from build123d import *

# Parameters (mm, degrees)
ESQUISSE1_R                  = 125
ESQUISSE1_W                  = 25
ESQUISSE1_H                  = 60
BOSS_EXTRU_1_DEPTH           = 5
ESQUISSE2_W                  = 5
ESQUISSE2_H                  = 30
BOSS_EXTRU_2_DEPTH           = 45
CONG_1_R                     = 15
ESQUISSE3_R                  = 6
ESQUISSE3_R_2                = 1.25
ENL_V_MAT_EXTRU_1_DEPTH      = 50
R_P_TITION_CIRCULAIRE1_COUNT = 3
ESQUISSE7_W                  = 24
ESQUISSE7_H                  = 37
BOSS_EXTRU_4_DEPTH           = 4.1
ESQUISSE8_R                  = 3
ENL_V_MAT_EXTRU_2_DEPTH      = 183.41436347
R_P_TITION_CIRCULAIRE2_COUNT = 3


with BuildPart() as part:
    # Esquisse1 → Boss.-Extru.1 (new body)
    with BuildSketch(Plane(origin=(0, 0, 0), x_dir=(1, 0, 0), z_dir=(0, 1, 0))):
        with Locations(Location((0, 0, 0), (0, 0, 270))):
            Circle(ESQUISSE1_R)
        with Locations((-100, 0)):
            Rectangle(ESQUISSE1_W, ESQUISSE1_H, mode=Mode.SUBTRACT)
        Polygon((82.230762114, 82.427857926), (30.269237886, 112.427857926), (17.769237886, 90.777222831), (69.730762114, 60.777222831), align=None, mode=Mode.SUBTRACT)
        Polygon((30.269237886, -112.427857926), (82.230762114, -82.427857926), (69.730762114, -60.777222831), (17.769237886, -90.777222831), align=None, mode=Mode.SUBTRACT)
    extrude(amount=BOSS_EXTRU_1_DEPTH)

    # Esquisse2 → Boss.-Extru.2 (add)
    with BuildSketch(Plane(origin=(0, 5, 0), x_dir=(1, 0, 0), z_dir=(0, 1, 0))):
        with Locations((-85, -15)):
            Rectangle(ESQUISSE2_W, ESQUISSE2_H)
        with Locations((-85, 15)):
            Rectangle(ESQUISSE2_W, ESQUISSE2_H)
        Polygon((69.730762114, 60.777222831), (67.230762114, 56.447095812), (15.269237886, 86.447095812), (17.769237886, 90.777222831), align=None)
        Polygon((17.769237886, -90.777222831), (15.269237886, -86.447095812), (67.230762114, -56.447095812), (69.730762114, -60.777222831), align=None)
    extrude(amount=BOSS_EXTRU_2_DEPTH)

    # Congé1
    cong_1_edges = [part.edges().sort_by_distance(p)[0] for p in [
        (-85, 50, -30),
        (-85, 50, 30),
        (68.480762114, 50, -58.612159322),
        (16.519237886, 50, -88.612159322),
        (16.519237886, 50, 88.612159322),
        (68.480762114, 50, 58.612159322),
    ]]
    fillet(cong_1_edges, radius=CONG_1_R)

    # Esquisse3 → Enlèv. mat.-Extru.1 (cut)
    with BuildSketch(Plane.ZY.offset(87.5)):
        with Locations((0, 20.5)):
            Circle(ESQUISSE3_R)
        with Locations((-7.75, 14.08)):
            Circle(ESQUISSE3_R_2)
        with Locations((-15.5, 27.5)):
            Circle(ESQUISSE3_R_2)
        with Locations((-7.75, 40.92)):
            Circle(ESQUISSE3_R_2)
        with Locations((7.75, 40.92)):
            Circle(ESQUISSE3_R_2)
        with Locations((15.5, 27.5)):
            Circle(ESQUISSE3_R_2)
        with Locations((7.75, 14.08)):
            Circle(ESQUISSE3_R_2)
    enl_v_mat_extru_1 = extrude(amount=-ENL_V_MAT_EXTRU_1_DEPTH, mode=Mode.SUBTRACT)

    # Répétition circulaire1: Enlèv. mat.-Extru.1 ×3 about axis
    r_p_tition_circulaire1_axis = Axis((0, 5, 0), (0, 1, 0))
    for i in range(1, R_P_TITION_CIRCULAIRE1_COUNT):
        add(enl_v_mat_extru_1.rotate(r_p_tition_circulaire1_axis, i * 360 / R_P_TITION_CIRCULAIRE1_COUNT), mode=Mode.SUBTRACT)

    # Esquisse7 → Boss.-Extru.4 (add)
    with BuildSketch(Plane(origin=(0, 5, 0), x_dir=(1, 0, 0), z_dir=(0, 1, 0))):
        with Locations((-70.5, 0)):
            Rectangle(ESQUISSE7_W, ESQUISSE7_H)
    boss_extru_4 = extrude(amount=BOSS_EXTRU_4_DEPTH)

    # Esquisse8 → Enlèv. mat.-Extru.2 (cut, through all)
    with BuildSketch(Plane(origin=(0, 5, 0), x_dir=(1, 0, 0), z_dir=(0, 1, 0))):
        with Locations(Location((-77.5, 24.303995394, 0), (0, 0, 270))):
            Circle(ESQUISSE8_R)
        with Locations(Location((-62.5, 24.303995394, 0), (0, 0, 270))):
            Circle(ESQUISSE8_R)
        with Locations(Location((-62.5, -24.303995394, 0), (0, 0, 90))):
            Circle(ESQUISSE8_R)
        with Locations(Location((-77.5, -24.303995394, 0), (0, 0, 90))):
            Circle(ESQUISSE8_R)
    enl_v_mat_extru_2 = extrude(amount=-ENL_V_MAT_EXTRU_2_DEPTH, mode=Mode.SUBTRACT)

    # Répétition circulaire2: Boss.-Extru.4, Enlèv. mat.-Extru.2 ×3 about axis
    r_p_tition_circulaire2_axis = Axis((0, 0, 0), (0, 1, 0))
    add([boss_extru_4.rotate(r_p_tition_circulaire2_axis, i * 360 / R_P_TITION_CIRCULAIRE2_COUNT) for i in range(1, R_P_TITION_CIRCULAIRE2_COUNT)])
    add([enl_v_mat_extru_2.rotate(r_p_tition_circulaire2_axis, i * 360 / R_P_TITION_CIRCULAIRE2_COUNT) for i in range(1, R_P_TITION_CIRCULAIRE2_COUNT)], mode=Mode.SUBTRACT)


solid = part.part
Source: CAD feature listing. Evaluate the final solid. Frame: model axes, mm. A direction names the side the tool comes from. Round coordinates to 2 decimals unless told otherwise and drop trailing zeros. Loops run counter-clockwise (first coordinate to the right, second up) from the corner with the lowest first, then second, coordinate; pieces in that order, holes last.
Q1. Mould query, pull axis X, two halves, no side actions, for faces 1 (the face through (36, 9.1, -61)), 2 (the face through (62, 3, -57)), 3 (the face through (5.5, 2.46, -124.88)), 4 (the face through (23.93, 2.46, 101.45)). Classes: pulls with the +X half, pulls with the -X half, needs draft (parallel to the pull), parting line crosses it, or undercut.
Q2. Ray query, line 1 (Y direction, x = -84.4, z = -7.75); line 2 (Y direction, x = -68, z = -45.5); line 3 (X direction, y = 47, z = 1). Return the intervals inside material, ascending.
Q3. Section A-A, the plane x = -77.5. Return loops of the section in (y, z).
Q4. Section B-B, the plane y = 20.5. Return loops of the section in (x, z), plus the area to 3 significant figures.
Q5. Section C-C, the plane z = -105. Return loops of the section in (x, y).
Q6. First-contact query: P1, Ø3, axis at y = 27.5, z = 15.5, coming from the +X side; P2, Ø12, axis at x = -96, y = 10, coming from the -Z side; P3, Ø5.5, axis at x = -85, y = 16.5, coming from the -Z side; P4, Ø5, axis at x = 52.3, z = 41.97, coming from the +Y side. Flat tips, straight axial feed; report the tip coordinate or a pass-through.
Q7. Access query for faces 5 (the face through (64.79, 45.49, 60.78)), 6 (the face through (29.474, 7.021, 50.533)), 7 (the face through (-85.035, 20.764, -5.994)), 8 (the face through (43.386, 30.206, -75.987)), 9 (the face through (20.206, 45.489, 86.443)). Directions: +Z, -Z, +X, -X, +Y, -Y. A direction counts if a zero-diameter tool reaches every point of the face in a straight line with its end or side. Return the directions, or none.
Q8. Section D-D, the plane z = -35. Return loops of the section in (x, y), plus the area to 3 significant figures.
Solutions:
1. face 1: needs draft
1. face 2: undercut
1. face 3: parting line crosses it
1. face 4: undercut
2. line 1: y = 0 to 12.83, 15.33 to 39.67, 42.17 to 50
2. line 2: y = 0 to 5
2. line 3: x = -87.5 to -82.5
3. outline: (0, -98.08) - (5, -98.08) - (5, -27.3) - (0, -27.3) - close; (0, -21.3) - (5, -21.3) - (5, -18.5) - (9.1, -18.5) - (9.1, 18.5) - (5, 18.5) - (5, 21.3) - (0, 21.3) - close; (0, 27.3) - (5, 27.3) - (5, 98.08) - (0, 98.08) - close
4. outline: (-87.5, -30) - (-82.5, -30) - (-82.5, -6) - (-87.5, -6) - close; (-87.5, 6) - (-82.5, 6) - (-82.5, 30) - (-87.5, 30) - close; (15.27, -86.45) - (17.77, -90.78) - (38.55, -78.78) - (36.05, -74.45) - close; (15.27, 86.45) - (36.05, 74.45) - (38.55, 78.78) - (17.77, 90.78) - close; (46.45, -68.45) - (48.95, -72.78) - (69.73, -60.78) - (67.23, -56.45) - close; (46.45, 68.45) - (67.23, 56.45) - (69.73, 60.78) - (48.95, 72.78) - close
4. area: 720 mm2
5. outline: (-67.82, 0) - (25.98, 0) - (25.98, 5) - (-67.82, 5) - close; (43.13, 0) - (67.82, 0) - (67.82, 5) - (43.13, 5) - close
6. P1: stops at x = -82.5
6. P2: stops at z = -83.87
6. P3: stops at z = -30
6. P4: passes through
7. face 5: +X, +Y
7. face 6: -X, +Y
7. face 7: +X, -X
7. face 8: +Y, -Y
7. face 9: +Z, -X, +Y
8. outline: (-120, 0) - (120, 0) - (120, 5) - (-120, 5) - close
8. area: 1,200 mm2
